Can you work these out from the model? Positions are in its coordinate system, mm. Face numbers are marked on the shaded views. A direction names the side the tool comes from. Coordinates: 2 decimals unless noted, no trailing zeros. Loops run counter-clockwise (first coordinate to the right, second up) from the corner with the lowest first, then second, coordinate; pieces in that order, holes last.
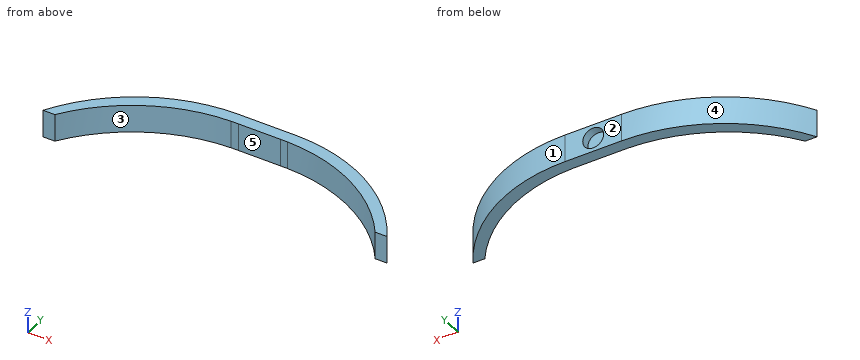
```python
from build123d import *

# Parameters (mm, degrees)
SKETCH1_W           = 15.24
SKETCH1_H           = 10.16
BOSS_EXTRUDE1_DEPTH = 4.3
BOSS_EXTRUDE2_DEPTH = 10.16
SKETCH3_R           = 3.81
CUT_EXTRUDE1_DEPTH  = 3


with BuildPart() as part:
    # Sketch1 → Boss-Extrude1 (new body)
    with BuildSketch(Plane(origin=(0, 0, 0), x_dir=(1, 0, 0), z_dir=(0, 1, 0))):
        Rectangle(SKETCH1_W, SKETCH1_H)
    extrude(amount=BOSS_EXTRUDE1_DEPTH)

    # Sketch2 → Boss-Extrude2 (add)
    with BuildSketch(Plane.XY.offset(5.08)):
        with BuildLine():
            Line((7.62, 4.3), (7.62, 0))
            Line((7.62, 0), (10.29, -0.020216112))
            ThreePointArc((10.29, -0.020216112), (37.444945357, -7.24175572), (58.419152196, -25.94))
            Line((58.419152196, -25.94), (62.719152196, -25.94))
            ThreePointArc((62.719152196, -25.94), (40.552491636, -3.80185252), (10.29, 4.3))
            Line((10.29, 4.3), (7.62, 4.3))
        make_face()
        with BuildLine():
            ThreePointArc((-10.29, 4.3), (-40.552491636, -3.80185252), (-62.719152196, -25.94))
            Line((-62.719152196, -25.94), (-58.419152196, -25.94))
            ThreePointArc((-58.419152196, -25.94), (-37.444945357, -7.24175572), (-10.29, -0.020216112))
            Line((-10.29, -0.020216112), (-7.62, 0))
            Line((-7.62, 0), (-7.62, 4.3))
            Line((-7.62, 4.3), (-10.29, 4.3))
        make_face()
    extrude(amount=-BOSS_EXTRUDE2_DEPTH)

    # Sketch3 → Cut-Extrude1 (cut)
    with BuildSketch(Plane(origin=(0, 4.3, 0), x_dir=(1, 0, 0), z_dir=(0, 1, 0))):
        Circle(SKETCH3_R)
    extrude(amount=-CUT_EXTRUDE1_DEPTH, mode=Mode.SUBTRACT)


solid = part.part
```
Item 1: Suppose I cut it at C-C, the plane z = 0. Please give me the cut outline in (x, y), plus the area to 3 significant figures.
Results are:
outline: (-62.72, -25.94) - (-58.42, -25.94) arc R60.57 cw to (-10.29, -0.02) - (-7.62, 0) - (7.62, 0) - (10.29, -0.02) arc R60.57 cw to (58.42, -25.94) - (62.72, -25.94) arc R60.57 ccw to (10.29, 4.3) - (3.81, 4.3) - (3.81, 1.3) - (-3.81, 1.3) - (-3.81, 4.3) - (-10.29, 4.3) arc R60.57 ccw to start
area: 586 mm2
Item 2: I'm going to push flat-ended pins straight in: P1, Ø3, axis at x = 30.5, z = 3, coming from the +Y side; P2, Ø4, axis at x = 20.5, z = -1.5, coming from the +Y side; P3, Ø5, axis at x = -1.5, z = -1, coming from the -Y side. Where does each tip first touch, or does it pass through?
Results are:
P1: stops at y = 1.34
P2: stops at y = 3.74
P3: stops at y = 0
Item 3: Suppose I cut it at A-A, the plane x = 0. Please give me the cut outline in (y, z).
Results are:
outline: (0, -5.08) - (4.3, -5.08) - (4.3, -3.81) - (1.3, -3.81) - (1.3, 3.81) - (4.3, 3.81) - (4.3, 5.08) - (0, 5.08) - close
Item 4: Suppose I cut it at D-D, the plane y = -1.5. Please give me the cut outline in (x, z).
Results are:
outline: (-36.15, -5.08) - (-22.12, -5.08) - (-22.12, 5.08) - (-36.15, 5.08) - close; (22.12, -5.08) - (36.15, -5.08) - (36.15, 5.08) - (22.12, 5.08) - close
Item 5: On a 3-axis mill with a long thin cutter (end or side, diameter ignored), from which of +Z, -Z, +X, -X, +Y, -Y can I reach the whole of each face in a straight line? I mean the marked faces 4 and 5. Say none if no direction works.
Results are:
face 4: +Z, -Z, -X, +Y
face 5: +Z, -Z, -Y
Item 6: I need wall thicknesses on line 1 along Z through (x, y) = (0, 3); line 2 along Y through (x, z) = (-7, 2.75); line 3 along X through (y, z) = (-18, 0.25). Which ranges of each line are inside material? Lowest first, please.
Results are:
line 1: z = -5.08 to -3.81, 3.81 to 5.08
line 2: y = 0 to 4.3
line 3: x = -57.24 to -51.81, 51.81 to 57.24
Item 7: Suppose I cut it at B-B, the plane y = -14.5. Please give me the cut outline in (x, z).
Results are:
outline: (-54.15, -5.08) - (-48.05, -5.08) - (-48.05, 5.08) - (-54.15, 5.08) - close; (48.05, -5.08) - (54.15, -5.08) - (54.15, 5.08) - (48.05, 5.08) - close
Item 8: We'd pull the mould along X, two halves only. Please class the marked faces 1, 2 and 3: +X half, -X half, draft (parallel to the pull), parting line (faces both ways), or undercut.
Results are:
face 1: +X half
face 2: draft
face 3: undercut
